Geometry: see drawing. Coordinates: mm, zero at the bounding-box minimum. Coordinates: 2 decimals unless noted, no trailing zeros. Order: outer loops, then holes, each group sorted by start corner. A loop starts at its lowest first (then second) coordinate and runs counter-clockwise, first axis right, second up. Notation, with made-up numbers: (77, 59.25) -> (82, 59.25) arc R26 ccw to (82, 81.25) -> close; hole circle Ø8 at (37, -20). An arc over 180 degrees is marked (long way). Write each question's results on one line, items separated by ' | '.
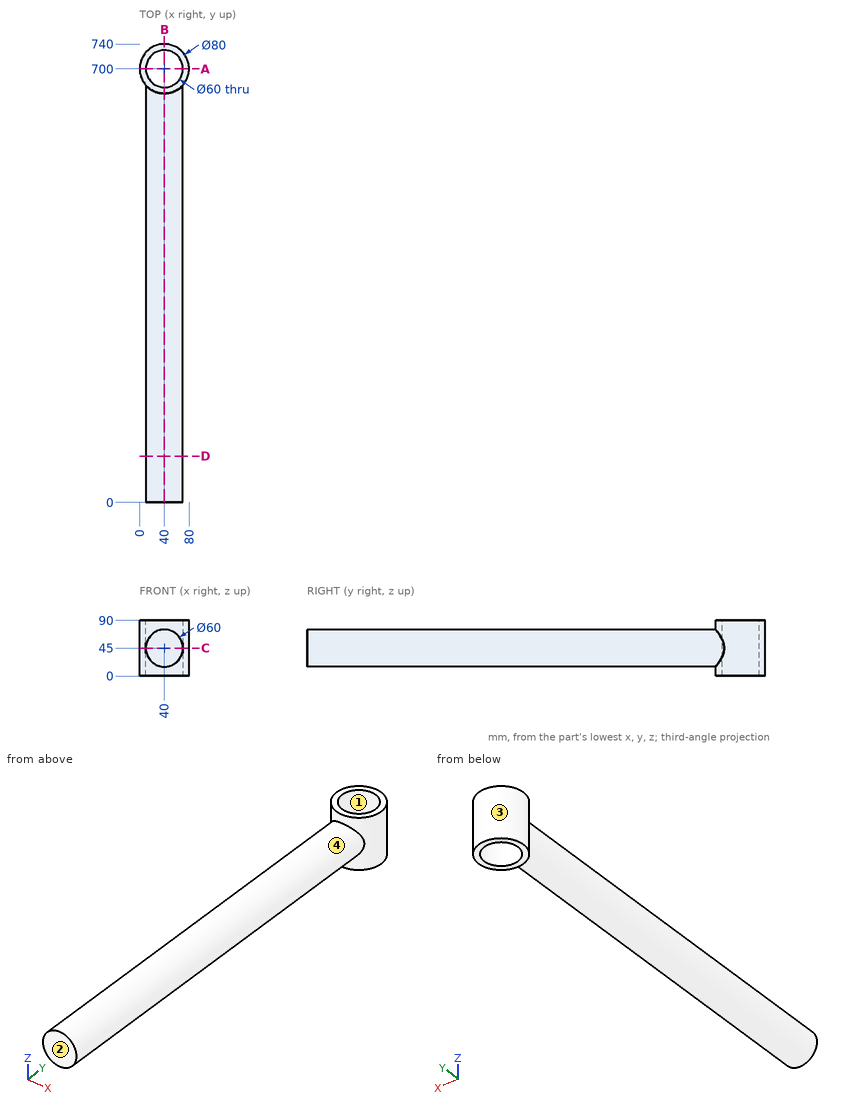
(1) Cut plane B-B, the plane x = 40. Return loops of the section in (y, z).
Return value:
outline: (0, 15) -> (660, 15) -> (660, 0) -> (670, 0) -> (670, 90) -> (660, 90) -> (660, 75) -> (0, 75) -> close; (730, 0) -> (740, 0) -> (740, 90) -> (730, 90) -> close
(2) Pin query (flat end, axial travel): P1, Ø8, axis at x = 12, z = 66.5, coming from the -Y side; P2, Ø1, axis at y = 290.5, z = 68.5, coming from the -X side; P3, Ø6, axis at x = 55.5, z = 43, coming from the +Y side. Return the tip coordinate at first contact, or that it passes through.
Return value:
P1: y = 668 | P2: x = 20.74 | P3: y = 738
(3) Line query: line 1 along Y through (x, z) = (38.5, 34); line 2 along X through (y, z) = (698, 44); line 3 along Y through (x, z) = (42.5, 78). Output: solid intervals per line, ascending. Write a range as from..to.
Return value:
line 1: 0..670.04, 729.96..739.97 | line 2: 0.05..10.07, 69.93..79.95 | line 3: 660.08..670.1, 729.9..739.92
(4) Cut plane D-D, the plane y = 74.5. Return loops of the section in (x, z), plus the area to 3 significant figures.
Return value:
outline: circle Ø60 at (40, 45) | area: 2,830 mm2
(5) Cut plane C-C, the plane z = 45. Return loops of the section in (x, y).
Return value:
outline: (10, 0) -> (70, 0) -> (70, 673.54) arc R40 ccw (long way) to (10, 673.54) -> close; hole circle Ø60 at (40, 700)
(6) Mould query, pull axis Y, two halves, no side actions, for the marked faces 1, 2, 3 and 4. Classes: +Y half, -Y half, draft (parallel to the pull), parting line (faces both ways), or undercut.
Return value:
face 1: undercut | face 2: -Y half | face 3: parting line | face 4: draft
(7) Cut plane A-A, the plane y = 700. Return loops of the section in (x, z).
Return value:
outline: (0, 0) -> (10, 0) -> (10, 90) -> (0, 90) -> close; (70, 0) -> (80, 0) -> (80, 90) -> (70, 90) -> close
